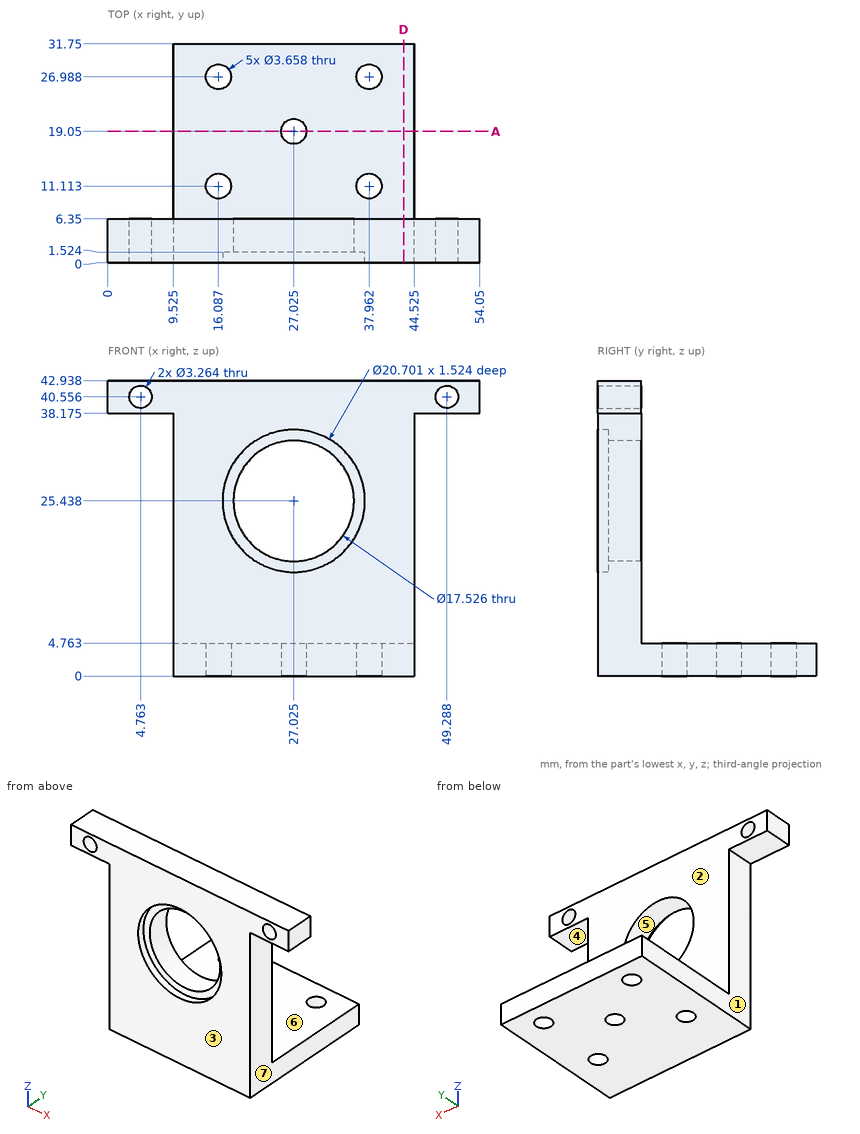
Here's the drawing with two shaded views (mm, measured from the low corner). I have some questions. A direction names the side the tool comes from. Coordinates: 2 decimals unless noted, no trailing zeros. Write each loop counter-clockwise with the first axis right and the second up, starting at its lowest first coordinate (ties: lowest second). Pieces come first, ordered by that corner, then holes. Notation, with made-up numbers: (29.25, 10.25) -> (65.25, 10.25) arc R27 cw to (65.25, 42.25) -> close; hole circle Ø2 at (85.5, -24.75). An arc over 180 degrees is marked (long way). Write item = value, one per line. Start each with the question number.
(1) I need wall thicknesses on line 1 (Z direction, x = 40, y = 11); line 2 (Y direction, x = 42, z = 21); line 3 (Z direction, x = 31.5, y = 5) (1 decimal). Which ranges of each line are inside material? Lowest first, please. Write a range as [from, to].
(2) Which directions (+Z, -Z, +X, -X, +Y, -Y) give clear straight access to the entire face, cutting with the end or side of a thin tool? Please do the marked faces 1, 2, 3 and 4.
(3) Will these pins go through, and if not, where does the flat tip stop? pin 1 (1.5 mm diameter, centred on y = 6, z = 13.5, fed in from +X) (1 decimal); pin 2 (5 mm diameter, centred on x = 51, y = 3.5, fed in from -Z) (1 decimal); pin 3 (5 mm diameter, centred on x = 11, z = 25.5, fed in from +Y).
(4) I want a section at A-A (y = 19.05). Please give me the cut outline in (x, z) (1 decimal), plus the area to 3 significant figures.
(5) I want a section at D-D (x = 43). Please give me the cut outline in (y, z).
(6) We'd pull the mould along X, two halves only. Please class the marked faces 5, 6 and 7: released by +X, released by -X, zero draft, split by the parting line, or undercut.
Result set:
q1.line_1 = [0, 4.76]
q1.line_2 = [0, 6.35]
q1.line_3 = [0, 17.9], [33, 42.9]
q2.face_1 = -Z, -X, +Y, -Y
q2.face_2 = +Z, +X, -X, +Y
q2.face_3 = +Z, -Z, +X, -X, -Y
q2.face_4 = -Z, +X, +Y, -Y
q3.pin_1 = 44.5
q3.pin_2 = 38.2
q3.pin_3 = 6.35
q4.outline = (9.5, 0) -> (25.2, 0) -> (25.2, 4.8) -> (9.5, 4.8) -> close; (28.9, 0) -> (44.5, 0) -> (44.5, 4.8) -> (28.9, 4.8) -> close
q4.area = 149 mm2
q5.outline = (0, 0) -> (31.75, 0) -> (31.75, 4.76) -> (6.35, 4.76) -> (6.35, 42.94) -> (0, 42.94) -> close
q6.face_5 = undercut
q6.face_6 = zero draft
q6.face_7 = released by +X
